Input: part model. Units: mm. Frame: model coordinates. Give positions to 0.01 mm unless a question says otherwise; leave off trailing zeros. Write each loop counter-clockwise with the first axis right and the second up, starting at its lowest first coordinate (ties: lowest second). Pieces come first, ordered by that corner, then holes. Notation, with made-up numbers: (-10, 86.25) -> (2, 86.25) arc R30 cw to (2, 114.25) -> close; hole circle Ø10 at (73.5, 5.25). An arc over 180 degrees is marked (long way). Return JSON: item names as keys, results as strings. Group by question number.
Item 1: Mould query, pull axis X, two halves, no side actions, for faces 1 (the face through (-13.415, -1.035, 0.761)), 2 (the face through (0, -10, 1)), 3 (the face through (-20, 0, 1)), 4 (the face through (15.99, 1.7, 0.76)). Classes: released by +X, released by -X, zero draft, split by the parting line, or undercut.
Item 2: Section C-C, the plane x = -10.5. Return loops of the section in (y, z), then the cut area to 3 significant figures.
Item 3: Section B-B, the plane z = 0.3. Count the separate pieces of the cut face and the enclosed holes in it, then the cut area to 3 significant figures.
Item 4: Section A-A, the plane x = 12.7. Return loops of the section in (y, z), then the cut area to 3 significant figures.
Item 5: Line query: line 1 (Y direction, x = 0, z = 1.4); line 2 (Y direction, x = 8, z = 0.95). Output: solid intervals per line, ascending. Write a range as [from, to].
from build123d import *

# Parameters (mm, degrees)
F0_W     = 40
F0_H     = 20
F0_W_2   = 2.54
F0_H_2   = 1.23
F0_H_3   = 2.54
F0_W_3   = 1.26
F1_DEPTH = 1.5
F2_D     = 1.5


with BuildPart() as f1:
    # F0 (on Top) → F1 (new body)
    with BuildSketch(Plane.XY):
        Rectangle(F0_W, F0_H)
        Polygon((-16.5, 1.73), (-16.5, 2.96), (-15.24, 2.96), (-12.7, 2.96), (-10.16, 2.96), (-7.62, 2.96), (-5.08, 2.96), (-2.54, 2.96), (0, 2.96), (2.54, 2.96), (5.08, 2.96), (7.62, 2.96), (10.16, 2.96), (12.7, 2.96), (15.24, 2.96), (16.5, 2.96), (16.5, 1.73), (16.5, -0.81), (16.5, -2.04), (15.24, -2.04), (12.7, -2.04), (10.16, -2.04), (7.62, -2.04), (5.08, -2.04), (2.54, -2.04), (0, -2.04), (-2.54, -2.04), (-5.08, -2.04), (-7.62, -2.04), (-10.16, -2.04), (-12.7, -2.04), (-15.24, -2.04), (-16.5, -2.04), (-16.5, -0.81), align=None, mode=Mode.SUBTRACT)
        with Locations((-11.43, 2.345)):
            Rectangle(F0_W_2, F0_H_2)
        with Locations((-13.97, 2.345)):
            Rectangle(F0_W_2, F0_H_2)
        with Locations((1.27, 0.46)):
            Rectangle(F0_W_2, F0_H_3)
        with Locations((-1.27, -1.425)):
            Rectangle(F0_W_2, F0_H_2)
        with Locations((13.97, -1.425)):
            Rectangle(F0_W_2, F0_H_2)
        with Locations((13.97, 2.345)):
            Rectangle(F0_W_2, F0_H_2)
        with Locations((-15.87, 0.46)):
            Rectangle(F0_W_3, F0_H_3)
        with Locations((6.35, 0.46)):
            Rectangle(F0_W_2, F0_H_3)
        with Locations((6.35, -1.425)):
            Rectangle(F0_W_2, F0_H_2)
        with Locations((3.81, -1.425)):
            Rectangle(F0_W_2, F0_H_2)
        with Locations((8.89, 0.46)):
            Rectangle(F0_W_2, F0_H_3)
        with Locations((1.27, -1.425)):
            Rectangle(F0_W_2, F0_H_2)
        with Locations((-8.89, 0.46)):
            Rectangle(F0_W_2, F0_H_3)
        with Locations((-3.81, -1.425)):
            Rectangle(F0_W_2, F0_H_2)
        with Locations((11.43, 2.345)):
            Rectangle(F0_W_2, F0_H_2)
        with Locations((-13.97, -1.425)):
            Rectangle(F0_W_2, F0_H_2)
        with Locations((8.89, 2.345)):
            Rectangle(F0_W_2, F0_H_2)
        with Locations((-3.81, 2.345)):
            Rectangle(F0_W_2, F0_H_2)
        with Locations((-6.35, 2.345)):
            Rectangle(F0_W_2, F0_H_2)
        with Locations((1.27, 2.345)):
            Rectangle(F0_W_2, F0_H_2)
        with Locations((3.81, 2.345)):
            Rectangle(F0_W_2, F0_H_2)
        with Locations((15.87, 0.46)):
            Rectangle(F0_W_3, F0_H_3)
        with Locations((-1.27, 2.345)):
            Rectangle(F0_W_2, F0_H_2)
        with Locations((-8.89, 2.345)):
            Rectangle(F0_W_2, F0_H_2)
        with Locations((6.35, 2.345)):
            Rectangle(F0_W_2, F0_H_2)
        with Locations((-3.81, 0.46)):
            Rectangle(F0_W_2, F0_H_3)
        with Locations((-8.89, -1.425)):
            Rectangle(F0_W_2, F0_H_2)
        with Locations((-13.97, 0.46)):
            Rectangle(F0_W_2, F0_H_3)
        with Locations((3.81, 0.46)):
            Rectangle(F0_W_2, F0_H_3)
        with Locations((-11.43, 0.46)):
            Rectangle(F0_W_2, F0_H_3)
        with Locations((-11.43, -1.425)):
            Rectangle(F0_W_2, F0_H_2)
        with Locations((11.43, -1.425)):
            Rectangle(F0_W_2, F0_H_2)
        with Locations((-6.35, 0.46)):
            Rectangle(F0_W_2, F0_H_3)
        with Locations((-1.27, 0.46)):
            Rectangle(F0_W_2, F0_H_3)
        with Locations((13.97, 0.46)):
            Rectangle(F0_W_2, F0_H_3)
        with Locations((11.43, 0.46)):
            Rectangle(F0_W_2, F0_H_3)
        with Locations((8.89, -1.425)):
            Rectangle(F0_W_2, F0_H_2)
        with Locations((-6.35, -1.425)):
            Rectangle(F0_W_2, F0_H_2)
        with Locations((15.87, -1.425)):
            Rectangle(F0_W_3, F0_H_2)
        with Locations((-15.87, -1.425)):
            Rectangle(F0_W_3, F0_H_2)
        with Locations((15.87, 2.345)):
            Rectangle(F0_W_3, F0_H_2)
        with Locations((-15.87, 2.345)):
            Rectangle(F0_W_3, F0_H_2)
    extrude(amount=F1_DEPTH)

    # F2 (through all)
    with Locations(Plane(origin=(0, 0, 0), x_dir=(1, 0, 0), z_dir=(0, 0, -1))):
        with Locations((12.7, -1.73), (12.7, 0.81), (15.24, 0.81), (15.24, -1.73), (10.16, -1.73), (10.16, 0.81), (7.62, 0.81), (7.62, -1.73), (5.08, -1.73), (5.08, 0.81), (2.54, 0.81), (2.54, -1.73), (0, -1.73), (0, 0.81), (-2.54, 0.81), (-2.54, -1.73), (-5.08, -1.73), (-5.08, 0.81), (-7.62, 0.81), (-7.62, -1.73), (-10.16, -1.73), (-10.16, 0.81), (-12.7, 0.81), (-12.7, -1.73), (-15.24, -1.73), (-15.24, 0.81)):
            Hole(F2_D / 2)


solid = f1.part
Answer below:
{
 "1": {"face 1": "undercut", "face 2": "zero draft", "face 3": "released by -X", "face 4": "undercut"},
 "2": {"outline": "(-10, 0) -> (-1.48, 0) -> (-1.48, 1.5) -> (-10, 1.5) -> close; (-0.14, 0) -> (1.06, 0) -> (1.06, 1.5) -> (-0.14, 1.5) -> close; (2.4, 0) -> (10, 0) -> (10, 1.5) -> (2.4, 1.5) -> close", "area": "26.0 mm2"},
 "3": {"separate pieces": "1", "enclosed holes": "26", "area": "754 mm2"},
 "4": {"outline": "(-10, 0) -> (-1.56, 0) -> (-1.56, 1.5) -> (-10, 1.5) -> close; (-0.06, 0) -> (0.98, 0) -> (0.98, 1.5) -> (-0.06, 1.5) -> close; (2.48, 0) -> (10, 0) -> (10, 1.5) -> (2.48, 1.5) -> close", "area": "25.5 mm2"},
 "5": {"line 1": "y = [-10, -1.56], [-0.06, 0.98], [2.48, 10]", "line 2": "y = [-10, -1.46], [-0.16, 1.08], [2.38, 10]"}
}
